Can you work these out from the model? Positions are in its coordinate system, mm. Coordinates: 2 decimals unless noted, no trailing zeros. Write each loop counter-clockwise with the first axis right and the second up, starting at its lowest first coordinate (ties: lowest second). Pieces come first, ordered by that corner, then holes. Notation, with made-up numbers: (84, 8.5) - (99, 8.5) arc R34 ccw to (99, 39.5) - close; hole circle Ø2 at (47, -15). An arc over 180 degrees is marked (long way). Use one line per item in the form item = value. Start each with the question number.
(1) For pin 1 Ø0.6 at (x, y) = (79, 1) entering from +Z; pin 2 Ø1 at (x, y) = (-94, 0.5) entering from +Z; pin 3 Ø2 at (x, z) = (98.75, 40.25) entering from +Y; pin 4 Ø1 at (x, y) = (3.5, 1) entering from -Z, each with a flat end and sliding along its axis, tell me the tip position at first contact or that it passes through.
(2) If we section it at B-B on z = -89.5: Please give me the cut outline in (x, y).
(3) If I drill on probe 1 along X at (y, z) = (1.6, -5); probe 2 along X at (y, z) = (0.9, 32.45); probe 3 along Z at (x, y) = (57.1, 0.6), over which ranges is the centre line in solid material (lowest first)? Write a range as from..to.
(4) If we section it at C-C on x = -24: Please give me the cut outline in (y, z), then the cut area to 3 significant figures.
(5) If we section it at A-A on y = 0.8: Give the number of separate pieces and of enclosed holes in the cut face, then the cut area to 3 significant figures.
```python
from build123d import *

# Parameters (mm, degrees)
BOSS_EXTRU_1_DEPTH                  = 2
ESQUISSE2_W                         = 28
ESQUISSE2_H                         = 45.5
ENL_V_MAT_EXTRU_1_DEPTH             = 157.584109453
BOSS_EXTRU_2_DEPTH                  = 2
ESQUISSE11_R                        = 1.6
ENL_V_MAT_EXTRU_2_DEPTH             = 157.584109453
CONG_7_R                            = 3
CONG_8_R                            = 25
DIAM_TRE_DU_PER_AGE_3_4_3_4_2_D     = 3.4
DIAM_TRE_DU_PER_AGE_3_4_3_4_2_DEPTH = 3
DIAM_TRE_DU_PER_AGE_3_4_3_4_2_TIP   = 1.021463052
D_GAGEMENT_M31_D                    = 3.4
D_GAGEMENT_M33_D                    = 3.4
D_GAGEMENT_M33_DEPTH                = 7
D_GAGEMENT_M33_TIP                  = 1.021463052
ENL_V_MAT_EXTRU_3_DEPTH             = 154.681644706
BOSS_EXTRU_3_DEPTH                  = 2
ESQUISSE40_R                        = 1.6
ENL_V_MAT_EXTRU_4_DEPTH             = 154.681644706
CONG_9_R                            = 3


with BuildPart() as part:
    # Esquisse1 → Boss.-Extru.1 (new body)
    with BuildSketch(Plane(origin=(0, 0, 0), x_dir=(1, 0, 0), z_dir=(0, 1, 0))):
        Polygon((-102.5, 59.178402592), (-102.5, -59.178402592), (0, -118.356805184), (102.5, -59.178402592), (102.5, 59.178402592), (0, 118.356805184), align=None)
    extrude(amount=BOSS_EXTRU_1_DEPTH)

    # Esquisse2 → Enlèv. mat.-Extru.1 (cut, through all)
    with BuildSketch(Plane(origin=(0, 2, 0), x_dir=(1, 0, 0), z_dir=(0, 1, 0))):
        with Locations((-85.5, -4.75)):
            Rectangle(ESQUISSE2_W, ESQUISSE2_H)
        with Locations((85.5, -4.75)):
            Rectangle(ESQUISSE2_W, ESQUISSE2_H)
    extrude(amount=-ENL_V_MAT_EXTRU_1_DEPTH, mode=Mode.SUBTRACT)

    # Esquisse10 → Boss.-Extru.2 (add)
    with BuildSketch(Plane(origin=(0, 2, 0), x_dir=(1, 0, 0), z_dir=(0, 1, 0))):
        with BuildLine():
            Line((89.6, 18), (89.6, 12))
            ThreePointArc((89.6, 12), (87.1, 9.5), (84.6, 12))
            Line((84.6, 12), (84.6, 18))
            Line((84.6, 18), (89.6, 18))
        make_face()
    boss_extru_2 = extrude(amount=-BOSS_EXTRU_2_DEPTH)

    # Esquisse11 → Enlèv. mat.-Extru.2 (cut, through all)
    with BuildSketch(Plane(origin=(0, 2, 0), x_dir=(1, 0, 0), z_dir=(0, 1, 0))):
        with Locations((83.75, 14)):
            Circle(ESQUISSE11_R)
        with Locations((90.45, 14)):
            Circle(ESQUISSE11_R)
    enl_v_mat_extru_2 = extrude(amount=-ENL_V_MAT_EXTRU_2_DEPTH, mode=Mode.SUBTRACT)

    # Symétrie4: Boss.-Extru.2, Enlèv. mat.-Extru.2 across plane
    add(boss_extru_2.mirror(Plane(origin=(0, 0, 0), x_dir=(0, 0, 1), z_dir=(1, 0, 0))))
    add(enl_v_mat_extru_2.mirror(Plane(origin=(0, 0, 0), x_dir=(0, 0, 1), z_dir=(1, 0, 0))), mode=Mode.SUBTRACT)

    # Congé7
    # the kernel refuses this fillet: 3 mm, written as the material it adds along each edge
    with BuildSketch(Plane(origin=(-89.6, 2, -18), x_dir=(0, 0, 1), z_dir=(0, -1, 0)), Plane(origin=(84.6, 2, -18), x_dir=(0, 0, 1), z_dir=(0, -1, 0))) as cong_7_piece_1:
        with BuildLine():
            CenterArc((3, 2.978856885), CONG_7_R, 180, 83.193609184)
            Line((0, 2.978856885), (-0.06, 2.978856885))
            Line((-0.06, 2.978856885), (-0.06, 0))
            Line((-0.06, 0), (0, -0.06))
            ThreePointArc((0, -0.06), (1.322227914, -0.06), (2.637344945, -0.059577138))
            Line((2.637344945, -0.059577138), (2.644455829, 0))
        make_face()
    extrude(amount=2)
    with BuildSketch(Plane(origin=(-71.5, 2, -18), x_dir=(0, 0, 1), z_dir=(0, -1, 0)), Plane(origin=(71.5, 2, -18), x_dir=(1, 0, 0), z_dir=(0, -1, 0)), Plane(origin=(-99.5, 2, -18), x_dir=(1, 0, 0), z_dir=(0, -1, 0)), Plane(origin=(-99.5, 2, 27.5), x_dir=(0, 0, -1), z_dir=(0, -1, 0)), Plane(origin=(99.5, 2, 27.5), x_dir=(-1, 0, 0), z_dir=(0, -1, 0)), Plane(origin=(99.5, 2, -18), x_dir=(0, 0, 1), z_dir=(0, -1, 0))) as cong_7_piece_2:
        with BuildLine():
            CenterArc((CONG_7_R, CONG_7_R), CONG_7_R, 180, 90)
            Line((0, CONG_7_R), (-CONG_7_R * 0.02, CONG_7_R))
            Line((-CONG_7_R * 0.02, CONG_7_R), (-CONG_7_R * 0.02, -CONG_7_R * 0.02))
            Line((-CONG_7_R * 0.02, -CONG_7_R * 0.02), (CONG_7_R, -CONG_7_R * 0.02))
            Line((CONG_7_R, -CONG_7_R * 0.02), (CONG_7_R, 0))
        make_face()
    extrude(amount=2)
    with BuildSketch(Plane(origin=(-84.6, 2, -18), x_dir=(1, 0, 0), z_dir=(0, -1, 0)), Plane(origin=(89.6, 2, -18), x_dir=(1, 0, 0), z_dir=(0, -1, 0))) as cong_7_piece_3:
        with BuildLine():
            CenterArc((2.978856885, 3), CONG_7_R, 186.806390816, 83.193609184)
            Line((0, 2.644455829), (-0.059577138, 2.637344945))
            ThreePointArc((-0.059577138, 2.637344945), (-0.06, 1.322227914), (-0.06, 0))
            Line((-0.06, 0), (0, -0.06))
            Line((0, -0.06), (2.978856885, -0.06))
            Line((2.978856885, -0.06), (2.978856885, 0))
        make_face()
    extrude(amount=2)
    with BuildSketch(Plane(origin=(-71.5, 2, 27.5), x_dir=(0, 0, -1), z_dir=(0, -1, 0)), Plane(origin=(71.5, 2, 27.5), x_dir=(1, 0, 0), z_dir=(0, -1, 0))) as cong_7_piece_4:
        with BuildLine():
            CenterArc((CONG_7_R, -CONG_7_R), CONG_7_R, 90, 90)
            Line((0, -CONG_7_R), (-CONG_7_R * 0.02, -CONG_7_R))
            Line((-CONG_7_R * 0.02, -CONG_7_R), (-CONG_7_R * 0.02, CONG_7_R * 0.02))
            Line((-CONG_7_R * 0.02, CONG_7_R * 0.02), (CONG_7_R, CONG_7_R * 0.02))
            Line((CONG_7_R, CONG_7_R * 0.02), (CONG_7_R, 0))
        make_face()
    extrude(amount=2)

    # Congé8
    cong_8_edges = [part.edges().sort_by_distance(p)[0] for p in [
        (0, 1, -118.356805184),
        (102.5, 1, -59.178402592),
        (102.5, 1, 59.178402592),
        (0, 1, 118.356805184),
        (-102.5, 1, 59.178402592),
        (-102.5, 1, -59.178402592),
    ]]
    fillet(cong_8_edges, radius=CONG_8_R)

    # Diamètre du perçage Ø3.4 (3.4)2
    with Locations(Plane(origin=(0, 2, 0), x_dir=(-1, 0, 0), z_dir=(0, 1, 0))):
        with Locations((0, -101), (0, 101)):
            Hole(DIAM_TRE_DU_PER_AGE_3_4_3_4_2_D / 2, depth=DIAM_TRE_DU_PER_AGE_3_4_3_4_2_DEPTH)
            with Locations((0, 0, -(DIAM_TRE_DU_PER_AGE_3_4_3_4_2_DEPTH + DIAM_TRE_DU_PER_AGE_3_4_3_4_2_TIP / 2))):  # 118° drill point
                Cone(0, DIAM_TRE_DU_PER_AGE_3_4_3_4_2_D / 2, DIAM_TRE_DU_PER_AGE_3_4_3_4_2_TIP, mode=Mode.SUBTRACT)

    # Dégagement M31 (through all)
    with Locations(Plane(origin=(0, 0, 0), x_dir=(-1, 0, 0), z_dir=(0, -1, 0))):
        with Locations((48.1, -23), (57.1, -23), (-57.1, -23), (-48.1, -23)):
            Hole(D_GAGEMENT_M31_D / 2)

    # Dégagement M33
    with Locations(Plane(origin=(0, 0, 0), x_dir=(-1, 0, 0), z_dir=(0, -1, 0))):
        with Locations((15.43813191, -105.113468551), (-15.43813191, -105.113468551), (-98.75, -40.25), (-98.75, -32.45), (-90.594469683, 27.994469683), (15.43813191, 104.789291724), (98.85, 27.55), (90.594469683, 27.994469683), (98.75, -40.25), (98.75, -32.45)):
            Hole(D_GAGEMENT_M33_D / 2, depth=D_GAGEMENT_M33_DEPTH)
            with Locations((0, 0, -(D_GAGEMENT_M33_DEPTH + D_GAGEMENT_M33_TIP / 2))):  # 118° drill point
                Cone(0, D_GAGEMENT_M33_D / 2, D_GAGEMENT_M33_TIP, mode=Mode.SUBTRACT)

    # Esquisse38 → Enlèv. mat.-Extru.3 (cut, through all)
    with BuildSketch(Plane(origin=(0, 2, 0), x_dir=(1, 0, 0), z_dir=(0, 1, 0))):
        Polygon((21.5, -18.5), (-8.5, -18.5), (-8.5, -29.5), (-21.5, -29.5), (-21.5, 15), (21.5, 15), align=None)
    extrude(amount=-ENL_V_MAT_EXTRU_3_DEPTH, mode=Mode.SUBTRACT)

    # Esquisse39 → Boss.-Extru.3 (add)
    with BuildSketch(Plane(origin=(0, 2, 0), x_dir=(1, 0, 0), z_dir=(0, 1, 0))):
        with BuildLine():
            Line((-8.5, -23.5), (-14.5, -23.5))
            ThreePointArc((-14.5, -23.5), (-17, -21), (-14.5, -18.5))
            Line((-14.5, -18.5), (-8.5, -18.5))
            ThreePointArc((-8.5, -18.5), (-6, -21), (-8.5, -23.5))
        make_face()
    extrude(amount=-BOSS_EXTRU_3_DEPTH)

    # Esquisse40 → Enlèv. mat.-Extru.4 (cut, through all)
    with BuildSketch(Plane(origin=(0, 2, 0), x_dir=(1, 0, 0), z_dir=(0, 1, 0))):
        with Locations((-12.5, -17.65)):
            Circle(ESQUISSE40_R)
        with Locations((-12.5, -24.35)):
            Circle(ESQUISSE40_R)
    extrude(amount=-ENL_V_MAT_EXTRU_4_DEPTH, mode=Mode.SUBTRACT)

    # Congé9
    # the kernel refuses this fillet: 3 mm, written as the material it adds along each edge
    with BuildSketch(Plane(origin=(21.5, 2, 18.5), x_dir=(-1, 0, 0), z_dir=(0, -1, 0)), Plane(origin=(21.5, 2, -15), x_dir=(0, 0, 1), z_dir=(0, -1, 0)), Plane(origin=(-21.5, 2, 29.5), x_dir=(0, 0, -1), z_dir=(0, -1, 0)), Plane(origin=(-8.5, 2, 29.5), x_dir=(-1, 0, 0), z_dir=(0, -1, 0))) as cong_9_piece_1:
        with BuildLine():
            CenterArc((CONG_9_R, CONG_9_R), CONG_9_R, 180, 90)
            Line((0, CONG_9_R), (-CONG_9_R * 0.02, CONG_9_R))
            Line((-CONG_9_R * 0.02, CONG_9_R), (-CONG_9_R * 0.02, -CONG_9_R * 0.02))
            Line((-CONG_9_R * 0.02, -CONG_9_R * 0.02), (CONG_9_R, -CONG_9_R * 0.02))
            Line((CONG_9_R, -CONG_9_R * 0.02), (CONG_9_R, 0))
        make_face()
    extrude(amount=2)
    with BuildSketch(Plane(origin=(-21.5, 2, -15), x_dir=(0, 0, 1), z_dir=(0, -1, 0))) as cong_9_piece_2:
        with BuildLine():
            CenterArc((CONG_9_R, -CONG_9_R), CONG_9_R, 90, 90)
            Line((0, -CONG_9_R), (-CONG_9_R * 0.02, -CONG_9_R))
            Line((-CONG_9_R * 0.02, -CONG_9_R), (-CONG_9_R * 0.02, CONG_9_R * 0.02))
            Line((-CONG_9_R * 0.02, CONG_9_R * 0.02), (CONG_9_R, CONG_9_R * 0.02))
            Line((CONG_9_R, CONG_9_R * 0.02), (CONG_9_R, 0))
        make_face()
    extrude(amount=2)
    with BuildSketch(Plane(origin=(-8.5, 2, 23.5), x_dir=(0, 0, 1), z_dir=(0, -1, 0))) as cong_9_piece_3:
        with BuildLine():
            CenterArc((2.978856885, 3), CONG_9_R, 186.806390816, 83.193609184)
            Line((0, 2.644455829), (-0.059577138, 2.637344945))
            ThreePointArc((-0.059577138, 2.637344945), (-0.06, 1.322227914), (-0.06, 0))
            Line((-0.06, 0), (0, -0.06))
            Line((0, -0.06), (2.978856885, -0.06))
            Line((2.978856885, -0.06), (2.978856885, 0))
        make_face()
    extrude(amount=2)


solid = part.part
```
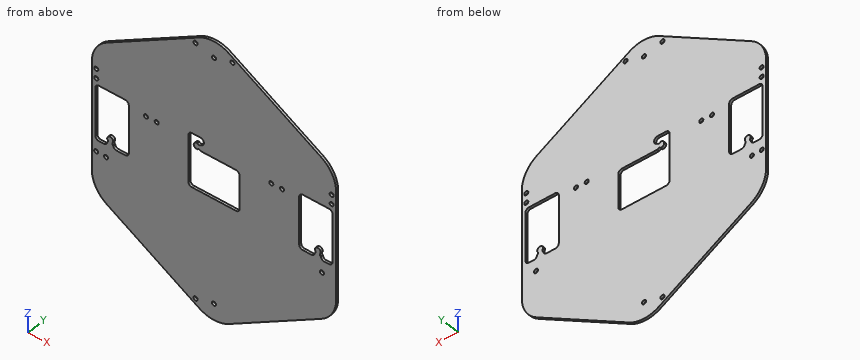
Reported:
q1.pin_1 = 72.92
q1.pin_2 = 63.95
q1.pin_3 = through
q1.pin_4 = -114.31
q2.outline = (-49.98, 0) - (49.98, 0) - (49.98, 2) - (-49.98, 2) - close
q3.probe_1 = -102.5..-99.5, -71.5..-21.5, 21.5..71.5, 99.5..102.5
q3.probe_2 = -102.5..-100.45, -97.05..97.05, 100.45..102.5
q3.probe_3 = -85.39..21.3, 24.7..85.39
q4.outline = (0, -104.5) - (2, -104.5) - (2, 104.5) - (0, 104.5) - close
q4.area = 418 mm2
q5.separate_pieces = 1
q5.enclosed_holes = 19
q5.area = 32,100 mm2
